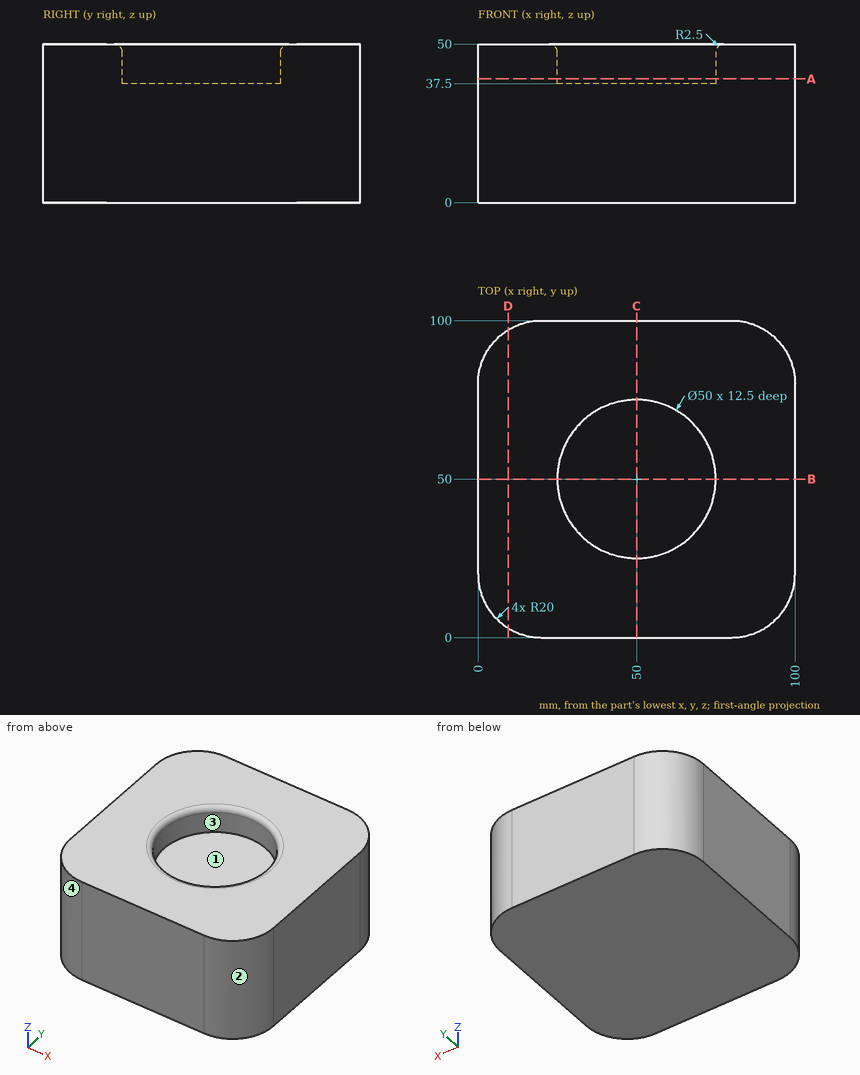
Study the drawing (mm; zero at the part's minimum x, y, z) and answer. Give positions to 0.01 mm unless a question says otherwise; leave off trailing zeros. Loops run counter-clockwise (first coordinate to the right, second up) from the corner with the lowest first, then second, coordinate; pieces in that order, holes last. Notation, with made-up numbers: M -20,32.25 L 10,32.25 A22 ccw 10,65.25 Z; hole C 77.25,0.5 d9. An arc over 180 degrees is marked long. One line per item, written item: value. Start each with the question number.
1. Find section B-B (y = 50). Give the vertices of the cut face in (x, z).
2. Find section D-D (x = 9.5). Give the vertices of the cut face in (y, z).
3. Find the intervals of material crossed by probe 1 along Y at (x, z) = (50, 43); probe 2 along X at (y, z) = (37, 47.5); probe 3 along Y at (x, z) = (35.5, 40.5), in increasing order.
4. Find section A-A (z = 39). Give the vertices of the cut face in (x, y), and give its area (3 significant figures).
5. Each of these flat-tipped pins is pushed along its axis until it touches: P1, Ø6, axis at x = 70.5, y = 43, coming from the -Z side; P2, Ø15, axis at x = 51, y = 52, coming from the +Z side; P3, Ø1, axis at y = 17.5, z = 41.5, coming from the -X side. Where does it stop, or does it pass through?
6. Determine the mould class of the marked faces 1, 2, 3 and 4 for opening direction X: released by +X, released by -X, zero draft, split by the parting line, or undercut.
Reported:
1. outline: M 0,0 L 100,0 L 100,50 L 77.5,50 A2.5 ccw 75,47.5 L 75,37.5 L 25,37.5 L 25,47.5 A2.5 ccw 22.5,50 L 0,50 Z
2. outline: M 2.98,0 L 97.02,0 L 97.02,50 L 2.98,50 Z
3. probe 1: y = 0 to 25, 75 to 100
3. probe 2: x = 0 to 28.65, 71.35 to 100
3. probe 3: y = 0 to 29.63, 70.37 to 100
4. outline: M 0,20 A20 ccw 20,0 L 80,0 A20 ccw 100,20 L 100,80 A20 ccw 80,100 L 20,100 A20 ccw 0,80 Z; hole C 50,50 d50
4. area: 7,690 mm²
5. P1: stops at z = 0
5. P2: stops at z = 37.5
5. P3: stops at x = 0.1
6. face 1: undercut
6. face 2: released by +X
6. face 3: undercut
6. face 4: released by -X
